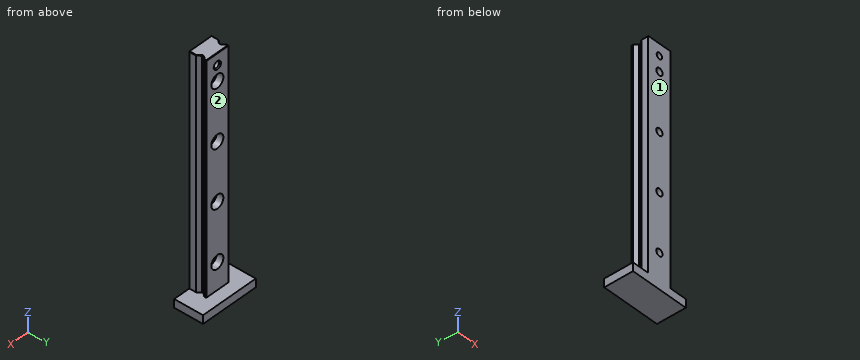
from build123d import *

# Parameters (mm, degrees)
P_IDAT_VYSUNUT_M1_DEPTH  = 140
SKICA2_W                 = 35
SKICA2_H                 = 17.21
P_IDAT_VYSUNUT_M2_DEPTH  = 5
SKICA3_R                 = 2.1
ODEBRAT_VYSUNUT_M1_DEPTH = 10
SKICA4_R                 = 4
ODEBRAT_VYSUNUT_M2_DEPTH = 4
SKICA5_R                 = 1.8
ODEBRAT_VYSUNUT_M3_DEPTH = 10
ZKOSEN_2_SIZE            = 0.25
ZKOSEN_3_SIZE            = 0.25
ZKOSEN_4_SIZE            = 0.6


with BuildPart() as part:
    # Skica1 → Přidat vysunutím1 (new body)
    with BuildSketch(Plane.XY):
        Polygon((0, 9), (1.749522731, 6.915), (1.749522731, 6.085), (0, 4), (0, 0), (15, 0), (15, 4), (13.250477269, 6.085), (13.250477269, 6.915), (15, 9), (15, 10), (0, 10), align=None)
    extrude(amount=P_IDAT_VYSUNUT_M1_DEPTH)

    # Skica2 → Přidat vysunutím2 (add)
    with BuildSketch(Plane(origin=(0, 0, 0), x_dir=(-1, 0, 0), z_dir=(0, 0, -1))):
        with Locations((-7.5, 8.605)):
            Rectangle(SKICA2_W, SKICA2_H)
    extrude(amount=-P_IDAT_VYSUNUT_M2_DEPTH)

    # Skica3 → Odebrat vysunutím1 (cut)
    with BuildSketch(Plane(origin=(0, 10, 0), x_dir=(1, 0, 0), z_dir=(0, 1, 0))):
        with Locations(Location((7.5, -124, 0), (0, 0, 180))):
            Circle(SKICA3_R)
        with Locations(Location((7.5, -89.666666667, 0), (0, 0, 180))):
            Circle(SKICA3_R)
        with Locations(Location((7.5, -55.333333333, 0), (0, 0, 180))):
            Circle(SKICA3_R)
        with Locations(Location((7.5, -21, 0), (0, 0, 180))):
            Circle(SKICA3_R)
    extrude(amount=-ODEBRAT_VYSUNUT_M1_DEPTH, mode=Mode.SUBTRACT)

    # Skica4 → Odebrat vysunutím2 (cut)
    with BuildSketch(Plane(origin=(0, 10, 0), x_dir=(1, 0, 0), z_dir=(0, 1, 0))):
        with Locations(Location((7.5, -124, 0), (0, 0, 180))):
            Circle(SKICA4_R)
        with Locations(Location((7.5, -89.67, 0), (0, 0, 180))):
            Circle(SKICA4_R)
        with Locations(Location((7.5, -55.34, 0), (0, 0, 180))):
            Circle(SKICA4_R)
        with Locations(Location((7.5, -21.01, 0), (0, 0, 180))):
            Circle(SKICA4_R)
    extrude(amount=-ODEBRAT_VYSUNUT_M2_DEPTH, mode=Mode.SUBTRACT)

    # Skica5 → Odebrat vysunutím3 (cut)
    with BuildSketch(Plane(origin=(0, 10, 0), x_dir=(1, 0, 0), z_dir=(0, 1, 0))):
        with Locations(Location((7.5, -133, 0), (0, 0, 180))):
            Circle(SKICA5_R)
    extrude(amount=-ODEBRAT_VYSUNUT_M3_DEPTH, mode=Mode.SUBTRACT)

    # Zkosení2
    zkosen_2_edges = [part.edges().sort_by_distance(p)[0] for p in [
        (15, 2, 140),
        (14.125238634, 5.0425, 140),
        (13.250477269, 6.5, 140),
        (14.125238634, 7.9575, 140),
        (15, 9.5, 140),
        (7.5, 10, 140),
        (0, 9.5, 140),
        (0.874761366, 7.9575, 140),
        (1.749522731, 6.5, 140),
        (0.874761366, 5.0425, 140),
        (0, 2, 140),
    ]]
    chamfer(zkosen_2_edges, length=ZKOSEN_2_SIZE)

    # Zkosení3
    zkosen_3_edges = [part.edges().sort_by_distance(p)[0] for p in [
        (15, 10, 72.375),
        (0, 10, 72.375),
    ]]
    chamfer(zkosen_3_edges, length=ZKOSEN_3_SIZE)

    # Zkosení4
    zkosen_4_edges = [part.edges().sort_by_distance(p)[0] for p in [
        (9.3, 10, 133),
    ]]
    chamfer(zkosen_4_edges, length=ZKOSEN_4_SIZE)


solid = part.part
CAD build for the part. Positions are in the model's coordinates, mm. Face numbers are marked on the shaded views. A direction names the side the tool comes from. Round coordinates to 2 decimals unless told otherwise and drop trailing zeros. Loops run counter-clockwise (first coordinate to the right, second up) from the corner with the lowest first, then second, coordinate; pieces in that order, holes last. Notation, with made-up numbers: M -21.75,30 L 5.25,30 A24 cw 5.25,63 Z; hole C 57,84.25 d3. An arc over 180 degrees is marked long. One line per question, with ' | ' between items. Start each with the question number.
Item 1: Cut at C-C, the plane x = 22. Write the cut outline in (y, z).
Item 2: Cut at D-D, the plane y = 2. Write the cut outline in (x, z), plus the area to 3 significant figures.
Item 3: Wall check: line 1 (Z direction, x = 7.5, y = 4.6); line 2 (Z direction, x = 7.5, y = 7.5); line 3 (Z direction, x = 23, y = 16). Give the ranges that are in metal, low to high.
Item 4: Cut at A-A, the plane z = 124. Write the cut outline in (x, y) (3 decimals), plus the area to 3 significant figures.
Item 5: Cut at B-B, the plane z = 30. Write the cut outline in (x, y) (3 decimals), plus the area to 3 significant figures.
Item 6: Pin check, flat tips, straight feed: pin 1 Ø12 at (x, z) = (18, 111.5) entering from +Y; pin 2 Ø5 at (y, z) = (11, 93) entering from +X; pin 3 Ø0.9 at (y, z) = (6.5, 100) entering from +X. Stop position of each tip, or through.
Item 7: Which spindle directions (+Z, -Z, +X, -X, +Y, -Y) get a long thin tool onto all of the face, cutting with end or side? Do the marked faces 1 and 2. Say none if no direction does.
Responses:
1) outline: M 0,0 L 17.21,0 L 17.21,5 L 0,5 Z
2) outline: M -10,0 L 25,0 L 25,5 L 15,5 L 15,139.75 L 14.75,140 L 0.25,140 L 0,139.75 L 0,5 L -10,5 Z; hole C 7.5,21 d4.2; hole C 7.5,55.33 d4.2; hole C 7.5,89.67 d4.2; hole C 7.5,124 d4.2; hole C 7.5,133 d3.6 | area: 2,130 mm²
3) line 1: z = 0 to 18.9, 23.1 to 53.23, 57.43 to 87.57, 91.77 to 121.9, 126.1 to 131.2, 134.8 to 140 | line 2: z = 0 to 17.01, 25.01 to 51.34, 59.34 to 85.67, 93.67 to 120, 128 to 131.2, 134.8 to 140 | line 3: z = 0 to 5
4) outline: M 0,0 L 5.4,0 L 5.4,6 L 3.5,6 L 3.5,10 L 0.25,10 L 0,9.75 L 0,9 L 1.75,6.915 L 1.75,6.085 L 0,4 Z; M 9.6,0 L 15,0 L 15,4 L 13.25,6.085 L 13.25,6.915 L 15,9 L 15,9.75 L 14.75,10 L 11.5,10 L 11.5,6 L 9.6,6 Z | area: 82.5 mm²
5) outline: M 0,0 L 15,0 L 15,4 L 13.25,6.085 L 13.25,6.915 L 15,9 L 15,9.75 L 14.75,10 L 0.25,10 L 0,9.75 L 0,9 L 1.75,6.915 L 1.75,6.085 L 0,4 Z | area: 140 mm²
6) pin 1: stops at y = 10 | pin 2: stops at x = 15 | pin 3: stops at x = 13.28
7) face 1: +Z, -Z, +X, -X, -Y | face 2: +Z, +X, -X, +Y
